```python
from build123d import *

# Parameters (mm, degrees)
F0_W     = 63.619988
F0_H     = 21
F1_DEPTH = 2.5


with BuildPart() as f1:
    # F0 (on Right) → F1 (new body)
    with BuildSketch(Plane.YZ):
        Polygon((0, 125), (0, 0), (75, 0), (75, 125), (71.19, 125), (71.19, 43.36109), (71.19, 3.81), (3.81, 3.81), (3.81, 121.19), (44.505585, 121.19), (47.69, 121.19), (50.19, 121.19), (50.19, 125), (44.505585, 125), align=None)
        Polygon((71.19, 3.81), (71.19, 43.36109), (26.69, 43.36109), (26.69, 95.11), (5.69, 95.11), (5.69, 116.11), (47.69, 116.11), (47.69, 121.19), (44.505585, 121.19), (3.81, 121.19), (3.81, 3.81), align=None)
        with Locations((37.5, 19.39)):
            Rectangle(F0_W, F0_H, mode=Mode.SUBTRACT)
        Polygon((50.19, 64.36109), (50.19, 121.19), (47.69, 121.19), (47.69, 116.11), (47.69, 64.36109), align=None)
    extrude(amount=F1_DEPTH)


solid = f1.part
```
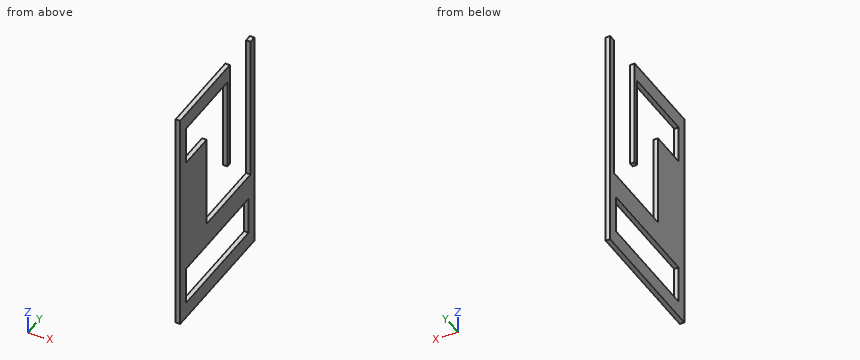
CAD build for the part. Positions are in the model's coordinates, mm. Give positions to 0.01 mm unless a question says otherwise; leave off trailing zeros. Order: outer loops, then holes, each group sorted by start corner. A loop starts at its lowest first (then second) coordinate and runs counter-clockwise, first axis right, second up.
(1) Saw through at C-C, the plane y = 31. Give the cut face in (x, z).
(2) Drill centre lines: L1, parallel to Z at x = 1.1, y = 47; L2, parallel to Y at x = 1.9, z = 65; L3, parallel to Z at x = 1.45, y = 11. Where is each one in solid material? Low to high.
(3) Saw through at D-D, the plane z = 52. Give the cut face in (x, y), then the cut area to 4 significant figures.
(4) Saw through at A-A, the plane y = 61. Give the cut face in (x, z), then the cut area to 3 significant figures.
(5) Saw through at B-B, the plane z = 107.5. Give the cut face in (x, y).
Results found:
1. outline: (0, 0) - (2.5, 0) - (2.5, 8.89) - (0, 8.89) - close; (0, 29.89) - (2.5, 29.89) - (2.5, 43.36) - (0, 43.36) - close; (0, 116.11) - (2.5, 116.11) - (2.5, 125) - (0, 125) - close
2. L1: z = 0 to 8.89, 29.89 to 43.36, 116.11 to 125
2. L2: y = 0 to 26.69, 47.69 to 50.19, 71.19 to 75
2. L3: z = 0 to 8.89, 29.89 to 95.11, 116.11 to 125
3. outline: (0, 0) - (2.5, 0) - (2.5, 26.69) - (0, 26.69) - close; (0, 71.19) - (2.5, 71.19) - (2.5, 75) - (0, 75) - close
3. area: 76.25 mm2
4. outline: (0, 0) - (2.5, 0) - (2.5, 8.89) - (0, 8.89) - close; (0, 29.89) - (2.5, 29.89) - (2.5, 43.36) - (0, 43.36) - close
4. area: 55.9 mm2
5. outline: (0, 0) - (2.5, 0) - (2.5, 5.69) - (0, 5.69) - close; (0, 47.69) - (2.5, 47.69) - (2.5, 50.19) - (0, 50.19) - close; (0, 71.19) - (2.5, 71.19) - (2.5, 75) - (0, 75) - close
